Verification items for the finished model (mm, model axes). Coordinates: 2 decimals unless noted, no trailing zeros. Write each loop counter-clockwise with the first axis right and the second up, starting at its lowest first coordinate (ties: lowest second). Pieces come first, ordered by that corner, then holes. Notation, with made-up numbers: (-0.5, 54) - (24.5, 54) arc R15 cw to (24.5, 79) - close; hole circle Ø11 at (-35.75, 24). An arc over 180 degrees is marked (long way). Use CSV: the item, a comma, the result in double quotes. Start each with the question number.
```python
from build123d import *

# Parameters (mm, degrees)
MODEL_W                 = 3
MODEL_H                 = 3
MODEL_R                 = 1.5
MODEL_H_2               = 9
SALIENTE_EXTRUIR1_DEPTH = 3


with BuildPart() as part:
    # Model → Saliente-Extruir1 (new body)
    with BuildSketch(Plane.XY):
        with BuildLine():
            Line((7.279746634, 294.056370254), (7.279746634, 240.056370254))
            ThreePointArc((7.279746634, 240.056370254), (8.597766118, 236.874389738), (11.779746634, 235.556370254))
            Line((11.779746634, 235.556370254), (47.779746634, 235.556370254))
            ThreePointArc((47.779746634, 235.556370254), (50.961727149, 236.874389738), (52.279746634, 240.056370254))
            Line((52.279746634, 240.056370254), (52.279746634, 294.056370254))
            ThreePointArc((52.279746634, 294.056370254), (50.961727149, 297.238350769), (47.779746634, 298.556370254))
            Line((47.779746634, 298.556370254), (11.779746634, 298.556370254))
            ThreePointArc((11.779746634, 298.556370254), (8.597766118, 297.238350769), (7.279746634, 294.056370254))
        make_face()
        with Locations((11.779746634, 240.056370254)):
            Rectangle(MODEL_W, MODEL_H, mode=Mode.SUBTRACT)
        with Locations((11.779746634, 249.056370254)):
            Rectangle(MODEL_W, MODEL_H, mode=Mode.SUBTRACT)
        with Locations((24.779746634, 241.306370254)):
            Circle(MODEL_R, mode=Mode.SUBTRACT)
        with Locations((11.779746634, 258.056370254)):
            Rectangle(MODEL_W, MODEL_H_2, mode=Mode.SUBTRACT)
        with Locations((34.779746634, 241.306370254)):
            Circle(MODEL_R, mode=Mode.SUBTRACT)
        with Locations((47.779746634, 240.056370254)):
            Rectangle(MODEL_W, MODEL_H, mode=Mode.SUBTRACT)
        with Locations((47.779746634, 249.056370254)):
            Rectangle(MODEL_W, MODEL_H, mode=Mode.SUBTRACT)
        with Locations((47.779746634, 258.056370254)):
            Rectangle(MODEL_W, MODEL_H_2, mode=Mode.SUBTRACT)
        with Locations((11.779746634, 267.056370254)):
            Rectangle(MODEL_W, MODEL_H, mode=Mode.SUBTRACT)
        with Locations((11.779746634, 276.056370254)):
            Rectangle(MODEL_W, MODEL_H_2, mode=Mode.SUBTRACT)
        with BuildLine():
            Line((28.279746634, 291.586497273), (28.279746634, 295.556370254))
            Line((28.279746634, 295.556370254), (31.279746634, 295.556370254))
            Line((31.279746634, 295.556370254), (31.279746634, 291.586497273))
            ThreePointArc((31.279746634, 291.586497273), (31.645772038, 291.220471869), (31.779746634, 290.720471869))
            Line((31.779746634, 290.720471869), (31.779746634, 288.256370254))
            Line((31.779746634, 288.256370254), (33.779746634, 286.256370254))
            Line((33.779746634, 286.256370254), (39.379746634, 286.256370254))
            ThreePointArc((39.379746634, 286.256370254), (39.733300024, 286.109923644), (39.879746634, 285.756370254))
            Line((39.879746634, 285.756370254), (39.879746634, 279.739428783))
            ThreePointArc((39.879746634, 279.739428783), (42.778382711, 271.556370254), (39.879746634, 263.373311725))
            Line((39.879746634, 263.373311725), (39.879746634, 246.006370254))
            ThreePointArc((39.879746634, 246.006370254), (39.733300024, 245.652816863), (39.379746634, 245.506370254))
            Line((39.379746634, 245.506370254), (30.579746634, 245.506370254))
            Line((30.579746634, 245.506370254), (30.579746634, 238.556370254))
            Line((30.579746634, 238.556370254), (28.979746634, 238.556370254))
            Line((28.979746634, 238.556370254), (28.979746634, 245.506370254))
            Line((28.979746634, 245.506370254), (20.179746634, 245.506370254))
            ThreePointArc((20.179746634, 245.506370254), (19.826193243, 245.652816863), (19.679746634, 246.006370254))
            Line((19.679746634, 246.006370254), (19.679746634, 263.369945552))
            ThreePointArc((19.679746634, 263.369945552), (16.778382711, 271.556370254), (19.679746634, 279.742794955))
            Line((19.679746634, 279.742794955), (19.679746634, 285.756370254))
            ThreePointArc((19.679746634, 285.756370254), (19.826193243, 286.109923644), (20.179746634, 286.256370254))
            Line((20.179746634, 286.256370254), (25.779746634, 286.256370254))
            Line((25.779746634, 286.256370254), (27.779746634, 288.256370254))
            Line((27.779746634, 288.256370254), (27.779746634, 290.720471869))
            ThreePointArc((27.779746634, 290.720471869), (27.91372123, 291.220471869), (28.279746634, 291.586497273))
        make_face(mode=Mode.SUBTRACT)
        with Locations((11.779746634, 285.056370254)):
            Rectangle(MODEL_W, MODEL_H, mode=Mode.SUBTRACT)
        with Locations((11.779746634, 294.056370254)):
            Rectangle(MODEL_W, MODEL_H, mode=Mode.SUBTRACT)
        with Locations((24.779746634, 289.806370254)):
            Circle(MODEL_R, mode=Mode.SUBTRACT)
        with Locations((20.779746634, 294.056370254)):
            Rectangle(MODEL_W, MODEL_H, mode=Mode.SUBTRACT)
        with Locations((47.779746634, 267.056370254)):
            Rectangle(MODEL_W, MODEL_H, mode=Mode.SUBTRACT)
        with Locations((47.779746634, 276.056370254)):
            Rectangle(MODEL_W, MODEL_H_2, mode=Mode.SUBTRACT)
        with Locations((34.779746634, 289.806370254)):
            Circle(MODEL_R, mode=Mode.SUBTRACT)
        with Locations((38.779746634, 294.056370254)):
            Rectangle(MODEL_W, MODEL_H, mode=Mode.SUBTRACT)
        with Locations((47.779746634, 285.056370254)):
            Rectangle(MODEL_W, MODEL_H, mode=Mode.SUBTRACT)
        with Locations((47.779746634, 294.056370254)):
            Rectangle(MODEL_W, MODEL_H, mode=Mode.SUBTRACT)
    extrude(amount=SALIENTE_EXTRUIR1_DEPTH)


solid = part.part
```
Q1. Scan lines: line 1 along X through (y, z) = (261, 2.95); line 2 along Y through (x, z) = (25, 1.15); line 3 along Y through (x, z) = (20.5, 1.45). Record each from-to range of solid material in increasing order. Write a range as from..to.
Q2. Release check for a two-part mould opening along X. For faces 1 (the flat face through (7.28, 267, 1)), 2 (the flat face through (21, 295.556, 1)), 3 (the flat face through (19, 260, 3)) record: released by +X, released by -X, zero draft, split by the parting line, or undercut.
Q3. Cross-section at D-D (x = 41.5). Record the cut outline in (y, z).
Q4. Cross-section at A-A (y = 260.5). Record the cut outline in (x, z).
Q5. Cross-section at B-B (y = 252). Record the cut outline in (x, z), plus the area to 3 significant figures.
Q6. Gauge pin test, flat end, axial feed: pin 1 (3.5 mm diameter, centred on x = 24.78, y = 241.31, fed in from +Z). Record the tip position at first contact, or that the pin passes through.
Q7. Cross-section at C-C (x = 47). State how many separate pieces and enclosed holes the cut face has, plus the area to 3 significant figures.
Reply:
1,line 1,"7.28..10.28, 13.28..19.68, 39.88..46.28, 49.28..52.28"
1,line 2,"235.56..239.82, 242.79..245.51, 286.26..288.32, 291.29..298.56"
1,line 3,"235.56..245.51, 286.26..292.56, 295.56..298.56"
2,face 1,"released by -X"
2,face 2,"undercut"
2,face 3,"zero draft"
3,outline,"(235.56, 0) - (265.93, 0) - (265.93, 3) - (235.56, 3) - close; (277.18, 0) - (298.56, 0) - (298.56, 3) - (277.18, 3) - close"
4,outline,"(7.28, 0) - (10.28, 0) - (10.28, 3) - (7.28, 3) - close; (13.28, 0) - (19.68, 0) - (19.68, 3) - (13.28, 3) - close; (39.88, 0) - (46.28, 0) - (46.28, 3) - (39.88, 3) - close; (49.28, 0) - (52.28, 0) - (52.28, 3) - (49.28, 3) - close"
5,outline,"(7.28, 0) - (19.68, 0) - (19.68, 3) - (7.28, 3) - close; (39.88, 0) - (52.28, 0) - (52.28, 3) - (39.88, 3) - close"
5,area,"74.4 mm^2"
6,pin 1,"z = 3"
7,separate pieces,"8"
7,enclosed holes,"0"
7,area,"90.0 mm^2"
